Answer from the drawing. Dimensions are ordinates in mm from the lowest x, y and z of the part. Round coordinates to 2 decimals unless told otherwise and drop trailing zeros. Loops run counter-clockwise (first coordinate to the right, second up) from the corner with the lowest first, then second, coordinate; pieces in that order, holes last.
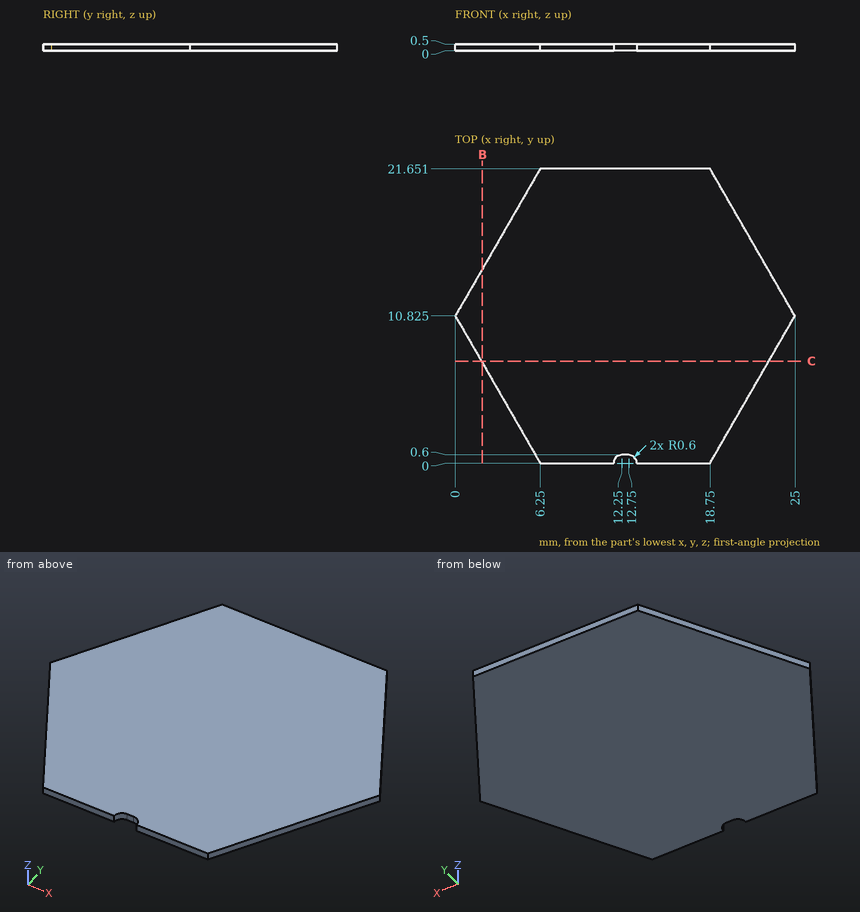
1. Consider probe 1 along X at (y, z) = (20.5, 0.4) (1 decimal); probe 2 along Y at (x, z) = (21, 0.35) (1 decimal); probe 3 along Y at (x, z) = (20, 0.4) (1 decimal). Determine where each line is inside the solid, lowest interval first.
Answer key:
probe 1: x = 5.6 to 19.4
probe 2: y = 3.9 to 17.8
probe 3: y = 2.2 to 19.5
2. Find section C-C (y = 7.5). Write down the section's boundary in (x, z).
Answer key:
outline: (1.92, 0) - (23.08, 0) - (23.08, 0.5) - (1.92, 0.5) - close
3. Find section B-B (x = 2). Write down the section's boundary in (y, z).
Answer key:
outline: (7.36, 0) - (14.29, 0) - (14.29, 0.5) - (7.36, 0.5) - close
